Autodesk Inventor part; units mm, degrees
ref_plane "YZ Plane" through (0, 0, 0) normal (1, 0, 0) x (0, 1, 0)
ref_plane "XZ Plane" through (0, 0, 0) normal (0, 1, 0) x (-1, 0, 0)
ref_plane "XY Plane" through (0, 0, 0) normal (0, 0, 1) x (1, 0, 0)
sketch "Sketch1" plane through (0, 0, 0) normal (0, 0, 1) x (1, 0, 0)
  line L0 (-64, 0) -> (-72, 0)
  line L1 (0, 37) -> (0, 24)
  line L2 (-72, 24) -> (-72, 37)
  line L3 (0, 0) -> (0, 24) construction
  line L4 (-72, 24) -> (0, 24)
  line L5 (-24, 22.0212) -> (-24, 32.5) construction
  line L6 (-24, 32.5) -> (-30, 32.5)
  line L7 (-30, 32.5) -> (-30, 28.5)
  line L8 (-30, 28.5) -> (-24, 28.5)
  line L9 (-24, 28.5) -> (-24, 32.5)
  line L10 (-30, 32.5) -> (-35, 32.5) construction
  line L11 (-22, 32.5) -> (-16, 32.5)
  line L12 (-16, 32.5) -> (-16, 28.5)
  line L13 (-16, 28.5) -> (-22, 28.5)
  line L14 (-22, 28.5) -> (-22, 32.5)
  line L15 (-14, 32.5) -> (-8, 32.5)
  line L16 (-8, 32.5) -> (-8, 28.5)
  line L17 (-8, 28.5) -> (-14, 28.5)
  line L18 (-14, 28.5) -> (-14, 32.5)
  line L19 (0, 24) -> (0, 37) construction
  line L20 (0, 37) -> (-91.064, 37) construction
  line L21 (0, 37) -> (-72, 37)
  line L22 (-72, 24) -> (-72, 37)
  line L23 (0, 24) -> (0, 37)
  line L24 (-72, 24) -> (-72, 30.5) construction
  line L25 (-72, 30.5) -> (-41.865, 30.5) construction
  line L26 (-64, 30.5) -> (-55.4, 30.5) construction
  line L27 (-55.4, 30.5) -> (-55.4, 35.5) construction
  line L28 (-55.4, 35.5) -> (-64, 30.5)
  line L29 (-55.4, 30.5) -> (-55.4, 25.5) construction
  line L30 (-64, 30.5) -> (-55.4, 25.5)
  line L31 (-32, 28.5) -> (-38, 28.5)
  line L32 (-38, 28.5) -> (-38, 32.5) construction
  line L33 (-38, 32.5) -> (-32, 32.5)
  line L34 (-32, 32.5) -> (-32, 28.5) construction
  line L35 (-38, 32.5) -> (-38, 28.5)
  line L36 (-32, 32.5) -> (-32, 28.5)
  line L37 (-40, 28.5) -> (-46, 28.5)
  line L38 (-46, 28.5) -> (-46, 32.5)
  line L39 (-46, 32.5) -> (-40, 32.5)
  line L40 (-40, 32.5) -> (-40, 28.5)
  line L41 (-55.4, 35.5) -> (-55.4, 32.5)
  line L42 (-55.4, 32.5) -> (-48, 32.5)
  line L43 (-48, 32.5) -> (-48, 28.5)
  line L44 (-48, 28.5) -> (-55.4, 28.5)
  line L45 (-55.4, 28.5) -> (-55.4, 25.5)
  point P0 (0, 0)
  point P1 (-137.4598, 47.0487)
  point P2 (-11, 28.5)
  point P3 (-11, 32.5)
  point P4 (-30, 30.5)
  point P5 (-32, 30.5)
  point P6 (-38, 30.5)
  point P7 (-40, 30.5)
  point P8 (-46, 30.5)
  point P9 (-48, 30.5)
  dimension "d3" = 0
  dimension "d4" = 0
  dimension "d8" = 24
  dimension "d14" = 6
  dimension "d19" = 6
  dimension "d20" = 4
  dimension "d21" = 6
  dimension "d22" = 2
  dimension "d23" = 2
  dimension "d33" = 8
  dimension "d36" = 28.5
  dimension "d37" = 13
  dimension "d38" = 4
  dimension "d39" = 8.6
  dimension "d40" = 5
  dimension "d41" = 5
  dimension "d42" = 6
  dimension "d43" = 4
  dimension "d44" = 2
  dimension "d45" = 6
  dimension "d46" = 2
  dimension "d47" = 3
  dimension "d48" = 7.4
extrude "Extrusion2" add sketch "Sketch1" along normal blind 1.5
properties part number "MS_R_Front_Green_v3"
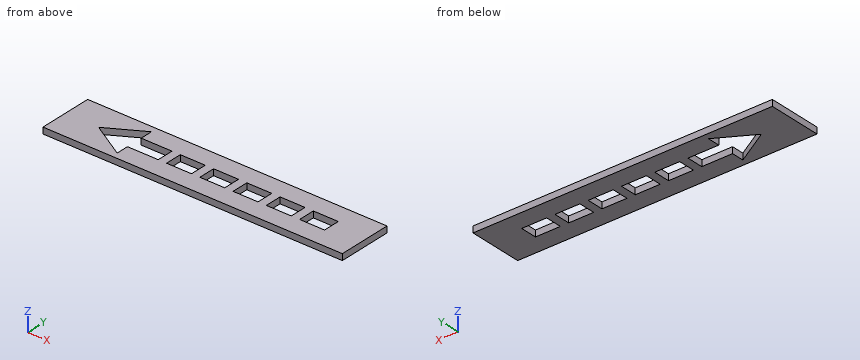
Build history of the part. All positions in model axes, mm. Give positions to 0.01 mm unless a question says otherwise; leave off trailing zeros. Loops run counter-clockwise (first coordinate to the right, second up) from the corner with the lowest first, then second, coordinate; pieces in that order, holes last. Notation, with made-up numbers: (-16.75, 71) -> (36.25, 71) arc R12 cw to (36.25, 80) -> close; hole circle Ø9 at (75.5, 27.25). An arc over 180 degrees is marked (long way). Answer in a Markdown table with one row per item.
Item 1: Slice it at B-B on x = -20.5. Write the cut outline in (y, z).
Findings below:
| item | result |
|---|---|
| outline | (24, 0) -> (28.5, 0) -> (28.5, 1.5) -> (24, 1.5) -> close; (32.5, 0) -> (37, 0) -> (37, 1.5) -> (32.5, 1.5) -> close |
Item 2: Slice it at C-C on z = 1.1. Give the number of separate pieces and of enclosed holes in the cut face, plus the area to 3 significant figures.
Findings below:
| item | result |
|---|---|
| separate pieces | 1 |
| enclosed holes | 6 |
| area | 743 mm² |
Item 3: Probe line 1 along Y through (x, z) = (-34.5, 1.1); line 2 along X through (y, z) = (33.25, 1.4); line 3 along X through (y, z) = (27, 0.3). List the from-to ranges inside material, lowest first. Write a range as [from, to].
Findings below:
| item | result |
|---|---|
| line 1 | y = [24, 28.5], [32.5, 37] |
| line 2 | x = [-72, -59.27], [-55.4, 0] |
| line 3 | x = [-72, -57.98], [-55.4, 0] |
Item 4: Slice it at A-A on y = 34.75. Write the cut outline in (x, z), plus the area to 3 significant figures.
Findings below:
| item | result |
|---|---|
| outline | (-72, 0) -> (-56.69, 0) -> (-56.69, 1.5) -> (-72, 1.5) -> close; (-55.4, 0) -> (0, 0) -> (0, 1.5) -> (-55.4, 1.5) -> close |
| area | 106 mm² |
